Can you work these out from the model? Positions are in its coordinate system, mm. Face numbers are marked on the shaded views. A direction names the side the tool comes from. Coordinates: 2 decimals unless noted, no trailing zeros. Loops run counter-clockwise (first coordinate to the right, second up) from the corner with the lowest first, then second, coordinate; pieces in that order, holes last. Notation, with made-up numbers: M 83.25,12 L 115.25,12 A12 cw 115.25,31 Z; hole C 42,44.5 d7. An arc over 180 degrees is marked long. Return JSON: item names as keys, results as strings. Group by question number.
```python
from build123d import *

# Parameters (mm, degrees)
F0_R     = 106.5
F0_R_2   = 75
F1_DEPTH = 30
F0_R_3   = 13.5
F2_DEPTH = 25


with BuildPart() as f1:
    # F0 (on Front) → F1 (new body)
    with BuildSketch(Plane.XZ):
        Circle(F0_R)
        Circle(F0_R_2, mode=Mode.SUBTRACT)
    extrude(amount=F1_DEPTH)

    # F0 (on Front) → F2 (join)
    with BuildSketch(Plane.XZ):
        Circle(F0_R_2)
        with BuildLine():
            ThreePointArc((-14.75, -48.930435), (-39.941343, -55.680435), (-21.5, -37.239092))
            ThreePointArc((-21.5, -37.239092), (-16.558657, -42.180435), (-14.75, -48.930435))
        make_face(mode=Mode.SUBTRACT)
        with BuildLine():
            ThreePointArc((-35.430435, -28.25), (-61.970434, -31.744057), (-37.239092, -21.5))
            ThreePointArc((-37.239092, -21.5), (-35.890437, -24.755943), (-35.430435, -28.25))
        make_face(mode=Mode.SUBTRACT)
        with BuildLine():
            ThreePointArc((13.5, -56.5), (-9.545942, -66.045942), (0, -43))
            ThreePointArc((0, -43), (9.545942, -46.954058), (13.5, -56.5))
        make_face(mode=Mode.SUBTRACT)
        with BuildLine():
            ThreePointArc((41.75, -48.930435), (21.5, -60.621778), (21.5, -37.239092))
            ThreePointArc((21.5, -37.239092), (35, -37.239092), (41.75, -48.930435))
        make_face(mode=Mode.SUBTRACT)
        with BuildLine():
            ThreePointArc((62.430435, -28.25), (45.436378, -41.289999), (37.239092, -21.5))
            ThreePointArc((37.239092, -21.5), (52.424492, -15.210001), (62.430435, -28.25))
        make_face(mode=Mode.SUBTRACT)
        with Locations((-56.5, 0)):
            Circle(F0_R_3, mode=Mode.SUBTRACT)
        with BuildLine():
            ThreePointArc((-35.430435, 28.25), (-35.890437, 24.755943), (-37.239092, 21.5))
            ThreePointArc((-37.239092, 21.5), (-61.970434, 31.744057), (-35.430435, 28.25))
        make_face(mode=Mode.SUBTRACT)
        with BuildLine():
            ThreePointArc((-14.75, 48.930435), (-16.558657, 42.180435), (-21.5, 37.239092))
            ThreePointArc((-21.5, 37.239092), (-39.941343, 55.680435), (-14.75, 48.930435))
        make_face(mode=Mode.SUBTRACT)
        with BuildLine():
            ThreePointArc((-18.75, 32.475953), (-9.705714, 36.222218), (0, 37.5))
            ThreePointArc((0, 37.5), (26.516504, 26.516504), (37.5, 0))
            ThreePointArc((37.5, 0), (36.222218, -9.705714), (32.475953, -18.75))
            ThreePointArc((32.475953, -18.75), (26.516504, -26.516504), (18.75, -32.475953))
            ThreePointArc((18.75, -32.475953), (9.705714, -36.222218), (0, -37.5))
            ThreePointArc((0, -37.5), (-9.705714, -36.222218), (-18.75, -32.475953))
            ThreePointArc((-18.75, -32.475953), (-26.516504, -26.516504), (-32.475953, -18.75))
            ThreePointArc((-32.475953, -18.75), (-36.222218, -9.705714), (-37.5, 0))
            ThreePointArc((-37.5, 0), (-36.222218, 9.705714), (-32.475953, 18.75))
            ThreePointArc((-32.475953, 18.75), (-26.516504, 26.516504), (-18.75, 32.475953))
        make_face(mode=Mode.SUBTRACT)
        with BuildLine():
            ThreePointArc((13.5, 56.5), (9.545942, 46.954058), (0, 43))
            ThreePointArc((0, 43), (-9.545942, 66.045942), (13.5, 56.5))
        make_face(mode=Mode.SUBTRACT)
    extrude(amount=F2_DEPTH)


solid = f1.part
```
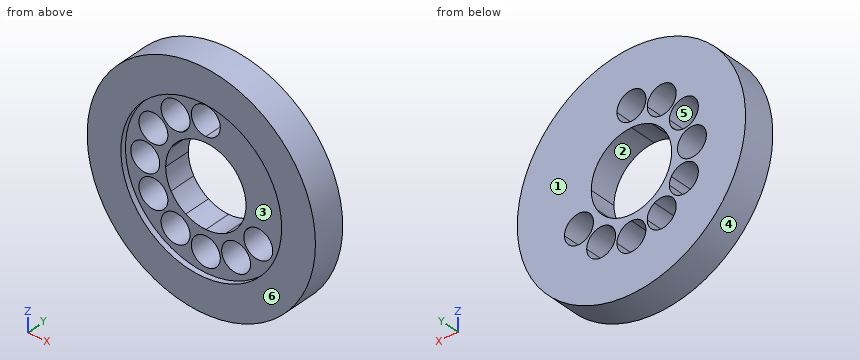
1) Suppose I cut it at B-B, the plane x = -56.5. List the corners of the cut face in (y, z) for me.
2) For pin 1 (24.5 mm diameter, centred on x = -28.25, z = 48.93, fed in from +Y); pin 2 (6 mm diameter, centred on x = -53.5, y = -21, fed in from +Z); pin 3 (1.5 mm diameter, centred on x = 14, y = -13, fed in from +Z); pin 4 (1.5 mm diameter, centred on x = -47, y = -25, fed in from -Z), each with a flat end and sliding along its axis, tell me the tip position at first contact or that it passes through.
3) For the marked faces 1, 2 and 3, which set-ups out of +Z, -Z, +X, -X, +Y, -Y let a thin tool reach every point of the face, with its end or its side?
4) Suppose I cut it at D-D, the plane x = 48.5. List the corners of the cut face in (y, z) for me, then the cut area to 3 significant figures.
5) Suppose I cut it at A-A, the plane y = -13. Give the number of separate pieces and of enclosed holes in the cut face, then the cut area to 3 significant figures.
6) Suppose I cut it at C-C, the plane z = -10.5. List the corners of the cut face in (x, y) for me.
7) If we mould it in two halves opening along X, with no side actions, what happens to the marked faces 4, 5 and 6? For each: +X half, -X half, draft (parallel to the pull), parting line (faces both ways), or undercut.
8) If I drill on line 1 (X direction, y = -24, z = 27.5); line 2 (X direction, y = -7, z = 6); line 3 (Z direction, x = 16.5, y = -5.25), over which ranges is the centre line in solid material (lowest first)? Write a range as from..to.
Returned:
{
 "1": {"outline": "M -30,-90.28 L 0,-90.28 L 0,-39.43 L -25,-39.43 L -25,-49.32 L -30,-49.32 Z; M -30,49.32 L -25,49.32 L -25,39.43 L 0,39.43 L 0,90.28 L -30,90.28 Z; M -25,-17.07 L 0,-17.07 L 0,-13.5 L -25,-13.5 Z; M -25,13.5 L 0,13.5 L 0,17.07 L -25,17.07 Z"},
 "2": {"pin 1": "passes through", "pin 2": "stops at z = 93.77", "pin 3": "stops at z = 105.67", "pin 4": "stops at z = -95.93"},
 "3": {"face 1": "+Z, -Z, +X, -X, +Y", "face 2": "+Y, -Y", "face 3": "-Y"},
 "4": {"outline": "M -30,-94.82 L 0,-94.82 L 0,-41.74 L -25,-41.74 L -25,-57.21 L -30,-57.21 Z; M -30,57.21 L -25,57.21 L -25,-14.76 L 0,-14.76 L 0,94.82 L -30,94.82 Z", "area": "4,440 mm²"},
 "5": {"separate pieces": "1", "enclosed holes": "10", "area": "26,100 mm²"},
 "6": {"outline": "M -105.98,-30 L -74.26,-30 L -74.26,-25 L -64.99,-25 L -64.99,0 L -105.98,0 Z; M -48.01,-25 L -36,-25 L -36,0 L -48.01,0 Z; M 36,-25 L 74.26,-25 L 74.26,-30 L 105.98,-30 L 105.98,0 L 36,0 Z"},
 "7": {"face 4": "parting line", "face 5": "undercut", "face 6": "draft"},
 "8": {"line 1": "x = -102.89..-62.41, -35.45..-25.5, 25.5..102.89", "line 2": "x = -106.33..-68.59, -44.41..-37.02, 37.02..106.33", "line 3": "z = -105.21..-55.58, -42.28..-33.67, 33.67..105.21"}
}
